Geometry check sheet. Reference: the model listing, model coordinates, mm. A direction names the side the tool comes from. Round coordinates to 2 decimals unless told otherwise and drop trailing zeros. Order: outer loops, then holes, each group sorted by start corner. A loop starts at its lowest first (then second) coordinate and runs counter-clockwise, first axis right, second up.
(1) Cross-section at A-A on x = -7.5. Enter the section's corners in (y, z).
(2) Thickness scan on L1, parallel to Z at x = -12.75, y = 11; L2, parallel to X at y = 3, z = 16; L3, parallel to Y at x = 1.5, z = 19.75. Record the ranges inside material, lowest first.
(3) Set-up check for faces 1 (the face through (-6, 34.586, 6)), 2 (the face through (-6, -6.914, 16)): record each of +Z, -Z, +X, -X, +Y, -Y from which the full face is reachable in a straight line by a thin tool's end or side.
(4) Cross-section at B-B on z = 20. Enter the section's corners in (x, y).
(5) Gauge pin test, flat ends, axial feed: P1, Ø2, axis at x = -6.5, y = 25, coming from the +Z side; P2, Ø10, axis at x = -10, z = 12, coming from the +Y side; P3, Ø6, axis at y = 10, z = 18.5, coming from the -X side; P4, Ø8, axis at x = -3, z = 17, coming from the +Y side. Record the tip position at first contact, or that the pin passes through.
from build123d import *

# Parameters (mm, degrees)
F0_W     = 22
F0_H     = 42
F1_DEPTH = 11.44
F2_W     = 0.5
F2_H     = 10
F3_DEPTH = 42
F4_W     = 0.5
F4_H     = 10
F5_DEPTH = 21.5


with BuildPart() as f1:
    # F0 (on Top) → F1 (new body)
    with BuildSketch(Plane.XY):
        with Locations((-6.227273, 13.585612)):
            Rectangle(F0_W, F0_H)
    extrude(amount=F1_DEPTH)

    # F2 (on face) → F3 (join)
    with BuildSketch(Plane.XZ.offset(7.414388)):
        with Locations((4.522727, 16.44)):
            Rectangle(F2_W, F2_H)
    extrude(amount=-F3_DEPTH)

    # F4 (on face) → F5 (join)
    with BuildSketch(Plane(origin=(4.272727, 0, 0), x_dir=(0, -1, 0), z_dir=(-1, 0, 0))):
        with Locations((7.164388, 16.44)):
            Rectangle(F4_W, F4_H)
    extrude(amount=F5_DEPTH)


solid = f1.part
Found:
1. outline: (-7.41, 0) - (34.59, 0) - (34.59, 11.44) - (-6.91, 11.44) - (-6.91, 21.44) - (-7.41, 21.44) - close
2. L1: z = 0 to 11.44
2. L2: x = 4.27 to 4.77
2. L3: y = -7.41 to -6.91
3. face 1: +Z, -Z, +X, -X, +Y
3. face 2: +Z, -X, +Y
4. outline: (-17.23, -7.41) - (4.77, -7.41) - (4.77, 34.59) - (4.27, 34.59) - (4.27, -6.91) - (-17.23, -6.91) - close
5. P1: stops at z = 11.44
5. P2: stops at y = 34.59
5. P3: stops at x = 4.27
5. P4: stops at y = -6.91
